Autodesk Inventor part; units mm, degrees
ref_plane "YZ Plane" through (0, 0, 0) normal (1, 0, 0) x (0, 1, 0)
ref_plane "XZ Plane" through (0, 0, 0) normal (0, 1, 0) x (-1, 0, 0)
ref_plane "XY Plane" through (0, 0, 0) normal (0, 0, 1) x (1, 0, 0)
sketch "Skizze1" plane through (0, 0, 0) normal (0, 1, 0) x (-1, 0, 0)
  line L0 (0, 0) -> (90, 0)
  line L1 (90, 0) -> (90, 20)
  line L2 (90, 20) -> (60, 20)
  line L3 (60, 20) -> (40, 107.7496)
  line L4 (40, 107.7496) -> (-40, 107.7496)
  line L5 (-40, 107.7496) -> (-60, 20)
  line L6 (-60, 20) -> (-90, 20)
  line L7 (-90, 20) -> (-90, 0)
  line L8 (-90, 0) -> (0, 0)
  dimension "d0" = 90
  dimension "d1" = 20
  dimension "d2" = 30
  dimension "d3" = 90
  dimension "d4" = 80
  dimension "d5" = 90
  dimension "d6" = 30
  dimension "d7" = 20
  dimension "d9" = 90
extrude "Extrusion1" add sketch "Skizze1" along normal blind 20
sketch "Skizze2" plane through (0, 20, 0) normal (0, 1, 0) x (1, 0, 0)
  line L0 (-60, -20) -> (-40, -107.7496) construction
  line L1 (-60, -20) -> (60, -20) construction
  line L2 (40.25, -107.7998) -> (-40.25, -107.7998)
  line L3 (-40.25, -107.7998) -> (-40.25, -19.9498)
  line L4 (-40.25, -19.9498) -> (40.25, -19.9498)
  line L5 (40.25, -19.9498) -> (40.25, -107.7998)
  line L6 (40.25, -107.7998) -> (-40.25, -19.9498) construction
  line L7 (-40.25, -107.7998) -> (40.25, -19.9498) construction
  point P0 (0, 0)
  point P1 (0, -63.8748)
  point P2 (0, -63.8748)
  dimension "d12" = 80.5
  dimension "d13" = 87.85
extrude "Extrusion2" cut sketch "Skizze2" against normal blind 10
sketch "Skizze3" plane through (0, 10, 0) normal (0, 1, 0) x (1, 0, 0)
  line L0 (40.25, -106.6528) -> (40, -107.7496)
  line L1 (40.25, -19.9498) -> (40.25, -106.6528)
  line L2 (-40.25, -19.9498) -> (40.25, -19.9498)
  line L3 (-40.25, -106.6528) -> (-40.25, -19.9498)
  line L4 (-40, -107.7496) -> (-40.25, -106.6528)
  line L5 (40, -107.7496) -> (-40, -107.7496)
  line L6 (30, -25.8013) -> (30, -100.8013)
  line L7 (30, -100.8013) -> (-30, -100.8013)
  line L8 (-30, -100.8013) -> (-30, -25.8013)
  line L9 (-30, -25.8013) -> (30, -25.8013)
  line L10 (30, -25.8013) -> (-30, -100.8013) construction
  line L11 (30, -100.8013) -> (-30, -25.8013) construction
  line L12 (-32.75, -100.2496) -> (-32.75, -27.4498) construction
  line L13 (-32.75, -27.4498) -> (32.75, -27.4498) construction
  line L14 (32.75, -27.4498) -> (32.75, -100.2496) construction
  line L15 (32.75, -100.2496) -> (-32.75, -100.2496) construction
  line L16 (-32.75, -63.8497) -> (-32.75, -40.3497) construction
  line L17 (-32.75, -63.8497) -> (-32.75, -87.3497) construction
  line L18 (-32.75, -87.3497) -> (32.75, -87.3497) construction
  line L19 (-32.75, -40.3497) -> (32.75, -40.3497) construction
  circle A0 centre (-32.75, -87.3497) radius 1.75
  circle A1 centre (-32.75, -40.3497) radius 1.75
  circle A2 centre (32.75, -40.3497) radius 1.75
  circle A3 centre (32.75, -87.3497) radius 1.75
  point P0 (0, 0)
  point P1 (0, -63.3013)
  point P2 (0, -63.3013)
  dimension "d16" = 75
  dimension "d17" = 60
  dimension "d18" = 7.5
  dimension "d19" = 23.5
  dimension "d20" = 23.5
  dimension "d21" = 3.5
  dimension "d22" = 3.5
  dimension "d23" = 3.5
  dimension "d24" = 3.5
extrude "Extrusion3" cut sketch "Skizze3" against normal blind 10 contours L6 L7 L8 L9 | A0 | A1 | A2 | A3
fillet "Rundung1" radius 5 4 edges at (-90, 10, 20) (90, 10, 20) (60, 10, 20) (-60, 10, 20)
fillet "Rundung2" radius 2 2 edges at (-40.25, 15, 19.9498) (40.25, 15, 19.9498)
sketch "Skizze4" plane through (-85, 0, 20) normal (0, 0, 1) x (1, 0, 0)
  line L0 (21.0114, 20) -> (21.0114, 0) construction
  line L1 (0, 20) -> (21.0114, 20) construction
  line L2 (0, 0) -> (0, 20) construction
  line L3 (0, 0) -> (21.0114, 0) construction
  line L4 (0, 0) -> (0, 20) construction
  line L5 (148.9886, 0) -> (148.9886, 20) construction
  line L6 (148.9886, 0) -> (170, 0) construction
  line L7 (170, 20) -> (170, 0) construction
  line L8 (148.9886, 20) -> (170, 20) construction
  line L9 (175, 20) -> (-5, 20) construction
  line L10 (159.4943, 20) -> (159.4943, 0) construction
  line L11 (148.9886, 10) -> (170, 10) construction
  line L12 (170, 20) -> (170, 0) construction
  line L13 (148.9886, 10) -> (159.4943, 20) construction
  line L14 (148.9886, 0) -> (148.9886, 20) construction
  line L15 (148.9886, 20) -> (159.4943, 10) construction
  line L16 (154.2415, 15) -> (159.4943, 15) construction
  line L17 (148.9886, 10) -> (159.4943, 0) construction
  line L18 (159.4943, 10) -> (148.9886, 0) construction
  line L19 (154.2415, 5) -> (159.4943, 5) construction
  line L20 (10.5057, 20) -> (10.5057, 0) construction
  line L21 (0, 20) -> (10.5057, 10) construction
  line L22 (10.5057, 20) -> (0, 10) construction
  line L23 (0, 10) -> (10.5057, 0) construction
  line L24 (10.5057, 10) -> (0, 0) construction
  line L25 (5.2528, 5) -> (10.5057, 5) construction
  line L26 (5.2528, 15) -> (10.5057, 15) construction
  point P0 (85, 0)
hole "Bohrung1" at (74.4943, 15, 20) at (74.4943, 5, 20) at (-74.4943, 15, 20) at (-74.4943, 5, 20) direction (0, 0, -1) diameter 4.5 end through all counterbore diameter 8 counterbore depth 4
chamfer "Fase1" distance 0.1 angle 45 8 edges at (-30, 10, 63.3013) (0, 10, 25.8013) (0, 10, 100.8013) (30, 10, 63.3013) (31, 10, 40.3497) (31, 10, 87.3497) (-34.5, 10, 40.3497) (-34.5, 10, 87.3497)
chamfer "Fase2" distance 1 angle 45 13 edges at (-40.25, 20, 64.3013) (-39.6642, 20, 20.5356) (0, 20, 19.9498) (39.6642, 20, 20.5356) (40.25, 20, 64.3013) (-49.6818, 20, 65.2708) (-74.4943, 20, 20) (-88.5355, 20, 18.5355) (-90, 20, 7.5) (49.6818, 20, 65.2708) (74.4943, 20, 20) (88.5355, 20, 18.5355) (90, 20, 7.5)
chamfer "Fase3" distance 0.1 angle 45 1 edges at (0, 10, 107.7496)
thread "Gewinde1"
thread "Gewinde2"
thread "Gewinde3"
thread "Gewinde4"
properties part number "Z-Motorhalter" material "Aluminium 6061"
The listing builds one solid part. Answer for the finished solid, in the listing's coordinates (mm). A direction names the side the tool comes from. Coordinates: 2 decimals unless noted, no trailing zeros. Loops run counter-clockwise (first coordinate to the right, second up) from the corner with the lowest first, then second, coordinate; pieces in that order, holes last. Notation, with made-up numbers: M 49.5,-39 L 86.5,-39 A15 cw 86.5,-21 Z; hole C -15.75,52.5 d4. An arc over 180 degrees is marked long. Answer in a Markdown table with one row per item.
1) Find section C-C (x = 10). Determine the outline of the cut face in (y, z), then the cut area to 3 significant figures.
Answers below:
| item | result |
|---|---|
| outline | M 0,0 L 20,0 L 20,18.95 L 19,19.95 L 10,19.95 L 10,25.7 L 9.9,25.8 L 0,25.8 Z; M 0,100.8 L 9.9,100.8 L 10,100.9 L 10,107.65 L 9.9,107.75 L 0,107.75 Z |
| area | 526 mm^2 |
2) Find section D-D (z = 55). Determine the outline of the cut face in (x, y).
Answers below:
| item | result |
|---|---|
| outline | M -52.02,0 L -30,0 L -30,9.9 L -30.1,10 L -40.25,10 L -40.25,19 L -41.25,20 L -51,20 L -52.02,19 Z; M 30,0 L 52.02,0 L 52.02,19 L 51,20 L 41.25,20 L 40.25,19 L 40.25,10 L 30.1,10 L 30,9.9 Z |
3) Find section A-A (x = 32.75). Determine the outline of the cut face in (y, z).
Answers below:
| item | result |
|---|---|
| outline | M 0,0 L 20,0 L 20,18.95 L 19,19.95 L 10,19.95 L 10,38.5 L 9.9,38.6 L 0,38.6 Z; M 0,42.1 L 9.9,42.1 L 10,42.2 L 10,85.5 L 9.9,85.6 L 0,85.6 Z; M 0,89.1 L 9.9,89.1 L 10,89.2 L 10,107.65 L 9.9,107.75 L 0,107.75 Z |
4) Which of the six approach directions +Z, -Z, +X, -X, +Y, -Y give full straight-line access (tool end or side, diameter ignored) to faces 1 (the flat face through (-74.6, 9.4, 20)), 2 (the cylindrical face through (70.53, 15.52, 17.97)), 3 (the flat face through (30, 5, 63))?
Answers below:
| item | result |
|---|---|
| face 1 | +Z, -X, +Y, -Y |
| face 2 | +Z |
| face 3 | +Y, -Y |
5) Find the intervals of material crossed by probe 1 along Z at (x, y) = (-32.75, 2.25); probe 2 along Y at (x, z) = (74.5, 8.5); probe 3 along X at (y, z) = (5, 5.25), in increasing order.
Answers below:
| item | result |
|---|---|
| probe 1 | 0 to 38.6, 42.1 to 85.6, 89.1 to 107.75 |
| probe 2 | 0 to 2.75, 7.25 to 12.75, 17.25 to 20 |
| probe 3 | -90 to -76.74, -72.24 to 72.24, 76.74 to 90 |
6) Find section B-B (y = 15). Count the separate pieces of the cut face and the enclosed holes in it, then the cut area to 3 significant figures.
Answers below:
| item | result |
|---|---|
| separate pieces | 3 |
| enclosed holes | 0 |
| area | 5,100 mm^2 |
7) Given pin 1 (3.5 mm diameter, centred on x = -74.49, y = 5, fed in from +Z); pin 2 (7 mm diameter, centred on y = 14.5, z = 63.5, fed in from +X); pin 3 (12 mm diameter, centred on x = -67.5, y = 11.5, fed in from -Z); pin 4 (4 mm diameter, centred on x = -76.5, y = 14, fed in from +Z), each flat-ended and moving along its own axis, determine where each tip first touches the part or whether it passes through.
Answers below:
| item | result |
|---|---|
| pin 1 | through |
| pin 2 | x = 50.88 |
| pin 3 | z = 0 |
| pin 4 | z = 20 |
8) Determine the mould class of faces 4 (the flat face through (76, 3, 16)), 5 (the conical face through (60.732, 19.285, 20.838)), 6 (the flat face through (90, 9, 8)) for opening direction Y: released by +Y, released by -Y, zero draft, split by the parting line, or undercut.
Answers below:
| item | result |
|---|---|
| face 4 | undercut |
| face 5 | released by +Y |
| face 6 | zero draft |
